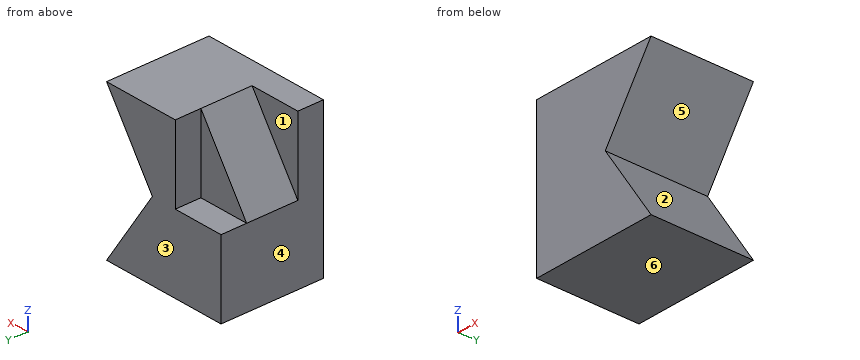
Autodesk Inventor part; units mm, degrees
ref_plane "YZ Plane" through (0, 0, 0) normal (1, 0, 0) x (0, 1, 0)
ref_plane "XZ Plane" through (0, 0, 0) normal (0, 1, 0) x (-1, 0, 0)
ref_plane "XY Plane" through (0, 0, 0) normal (0, 0, 1) x (1, 0, 0)
sketch "Sketch3" plane through (0, 0, 0) normal (0, 0, 1) x (1, 0, 0)
  line L0 (0, 0) -> (-10, 0)
  line L1 (-25, 0) -> (-25, 5)
  line L2 (-25, 5) -> (-15, 5)
  line L3 (-15, 5) -> (-15, 20)
  line L4 (-15, 20) -> (-10, 20)
  line L5 (0, 20) -> (0, 0)
  line L6 (0, 20) -> (-10, 20)
  line L7 (-10, 20) -> (-10, 0)
  line L8 (-10, 20) -> (0, 20)
  line L9 (-10, 0) -> (-25, 0)
  line L10 (-25, 5) -> (-25, 20)
  line L11 (-25, 20) -> (-15, 20)
  dimension "d12" = 25
  dimension "d13" = 5
  dimension "d14" = 10
  dimension "d15" = 15
  dimension "d16" = 15
  dimension "d19" = 10
extrude "Extrusion1" add sketch "Sketch3" along normal blind 15 contours L9 L1 L2 L3 L4 L7
extrude "Extrusion2" add sketch "Sketch3" against normal blind 15 contours L9 L1 L2 L3 L4 L7 | L3 L2 L10 L11
sketch "Sketch5" plane through (-25, 20, -15) normal (0, 1, 0) x (1, 0, 0)
  line L0 (15, 0) -> (15, -30)
  line L1 (15, 0) -> (15, -30)
  line L2 (15, -30) -> (25, -30)
  line L3 (25, -30) -> (15, -15)
  line L4 (15, 0) -> (25, 0)
  line L5 (25, 0) -> (15, -15)
  point P0 (25, -15)
  dimension "d24" = 10
  dimension "d25" = 10
extrude "Extrusion4" add sketch "Sketch5" against normal blind 20
sketch "Sketch6" plane through (-25, 5, 15) normal (0, 1, 0) x (1, 0, 0)
  line L0 (0, 15) -> (0, 0)
  line L1 (10, 15) -> (0, 15)
  line L2 (0, 15) -> (10, 0)
  line L3 (10, 15) -> (0, 15)
  line L4 (10, 0) -> (10, 15)
  point P0 (25, 15)
extrude "Extrusion5" add sketch "Sketch6" along normal blind 10
Could you check a few things on this model? Use its own coordinates, in mm. Face numbers are marked on the shaded views. A direction names the side the tool comes from. Give positions to 0.01 mm unless a question says otherwise; leave off trailing zeros. Order: outer loops, then holes, each group sorted by start corner. A loop starts at its lowest first (then second) coordinate and runs counter-clockwise, first axis right, second up.
Q1. Suppose I cut it at B-B, the plane z = 6.75. Write out the boundary of the cut face in (x, y).
Q2. If I drill on line 1 along Z through (x, y) = (-3, 3.25); line 2 along Z through (x, y) = (-23.5, 16.5); line 3 along X through (y, z) = (18.25, 6), over which ranges is the centre line in solid material (lowest first)?
Q3. For the marked faces 1, 2 and 3, which set-ups out of +Z, -Z, +X, -X, +Y, -Y let a thin tool reach every point of the face, with its end or its side?
Q4. Suppose I cut it at D-D, the plane y = 3.5. Write out the boundary of the cut face in (x, z).
Q5. Suppose I cut it at A-A, the plane x = -5.5. Write out the boundary of the cut face in (y, z), and give its area (3 significant figures).
Q6. I'm going to push flat-ended pins straight in: P1, Ø2.5, axis at x = -22.5, y = 18, coming from the +Z side; P2, Ø5, axis at y = 17.5, z = -3, coming from the +X side; P3, Ø4, axis at x = -6, z = -3.5, coming from the -Y side; P4, Ø5.5, axis at y = 18, z = 8.5, coming from the -X side. Where does each tip first touch, or does it pass through?
Q7. We'd pull the mould along Z, two halves only. Please class the marked faces 4, 5 and 6: +Z half, -Z half, draft (parallel to the pull), parting line (faces both ways), or undercut.
Q8. Suppose I cut it at C-C, the plane x = -22.5. Write out the boundary of the cut face in (y, z), and give its area (4 significant figures).
Solution:
1. outline: (-25, 0) - (-5.5, 0) - (-5.5, 20) - (-15, 20) - (-15, 15) - (-20.5, 15) - (-20.5, 5) - (-25, 5) - close
2. line 1: z = -15 to -10.5, 10.5 to 15
2. line 2: z = -15 to 0
2. line 3: x = -15 to -6
3. face 1: +Z, -X, +Y
3. face 2: +X, +Y, -Y
3. face 3: +Z, -Z, +X, -X, +Y
4. outline: (-25, -15) - (0, -15) - (-10, 0) - (0, 15) - (-25, 15) - close
5. outline: (0, -15) - (20, -15) - (20, -6.75) - (0, -6.75) - close; (0, 6.75) - (20, 6.75) - (20, 15) - (0, 15) - close
5. area: 330 mm2
6. P1: stops at z = 0
6. P2: stops at x = -6.33
6. P3: stops at y = 0
6. P4: stops at x = -15
7. face 4: draft
7. face 5: undercut
7. face 6: -Z half
8. outline: (0, -15) - (20, -15) - (20, 0) - (15, 0) - (15, 3.75) - (5, 3.75) - (5, 15) - (0, 15) - close
8. area: 412.5 mm2
